Could you check a few things on this model? Use its own coordinates, in mm. A direction names the side the tool comes from. Coordinates: 2 decimals unless noted, no trailing zeros. Loops run counter-clockwise (first coordinate to the right, second up) from the corner with the lowest first, then second, coordinate; pieces in that order, holes last.
from build123d import *

# Parameters (mm, degrees)
F0_R      = 2.0955
F0_R_2    = 4.826
F1_DEPTH  = 12.7
F2_R      = 2.0955
F3_DEPTH  = 15.875
F4_R      = 5.7785
F5_DEPTH  = 1.4478
F6_R      = 2.413
F7_DEPTH  = 31.75
F8_R      = 3.96875
F9_DEPTH  = 4.7498
F10_R     = 1.5875
F10_R_2   = 2.0066
F11_DEPTH = 9.525


with BuildPart() as f1:
    # F0 (on Top) → F1 (new body)
    with BuildSketch(Plane.XY):
        with BuildLine():
            Line((33.3375, -18.796), (33.3375, 18.796))
            Line((33.3375, 18.796), (-33.3375, 18.796))
            Line((-33.3375, 18.796), (-33.3375, 9.9949))
            Line((-33.3375, 9.9949), (-20.271096, 9.9949))
            ThreePointArc((-20.271096, 9.9949), (4.938511, -9.285687), (-21.315194, 8.5471))
            Line((-21.315194, 8.5471), (-33.3375, 8.5471))
            Line((-33.3375, 8.5471), (-33.3375, -18.796))
            Line((-33.3375, -18.796), (33.3375, -18.796))
        make_face()
        with Locations((-21.7805, -13.843)):
            Circle(F0_R, mode=Mode.SUBTRACT)
        with Locations((25.8699, -5.461)):
            Circle(F0_R_2, mode=Mode.SUBTRACT)
        with Locations((6.0325, 13.843)):
            Circle(F0_R, mode=Mode.SUBTRACT)
    extrude(amount=F1_DEPTH)

    # F2 (on face) → F3 (cut)
    with BuildSketch(Plane.YZ.offset(33.3375)):
        with Locations((-13.4874, 6.35)):
            Circle(F2_R)
        with Locations((13.4874, 6.35)):
            Circle(F2_R)
    extrude(amount=-F3_DEPTH, mode=Mode.SUBTRACT)

    # F4 (on face) → F5 (cut)
    with BuildSketch(Plane(origin=(0, 0, 0), x_dir=(1, 0, 0), z_dir=(0, 0, -1))):
        with Locations((25.8699, 5.461)):
            Circle(F4_R)
    extrude(amount=-F5_DEPTH, mode=Mode.SUBTRACT)

    # F6 (on face) → F7 (cut)
    with BuildSketch(Plane(origin=(0, 18.796, 0), x_dir=(-1, 0, 0), z_dir=(0, 1, 0))):
        with Locations((26.9875, 6.35)):
            Circle(F6_R)
    extrude(amount=-F7_DEPTH, mode=Mode.SUBTRACT)

    # F8 (on face) → F9 (cut)
    with BuildSketch(Plane(origin=(0, 18.796, 0), x_dir=(-1, 0, 0), z_dir=(0, 1, 0))):
        with Locations((26.9875, 6.35)):
            Circle(F8_R)
    extrude(amount=-F9_DEPTH, mode=Mode.SUBTRACT)

    # F10 (on face) → F11 (cut)
    with BuildSketch(Plane(origin=(0, 18.796, 0), x_dir=(-1, 0, 0), z_dir=(0, 1, 0))):
        with Locations((19.80565, 6.35)):
            Circle(F10_R)
        with Locations((0.75565, 6.35)):
            Circle(F10_R_2)
    extrude(amount=-F11_DEPTH, mode=Mode.SUBTRACT)


solid = f1.part
(1) Imagine slicing it at B-B, the plane y = 3.5. Write out the boundary of the cut face in (x, z), and give its area (3 significant figures).
Answers:
outline: (-33.34, 0) - (-23.42, 0) - (-23.42, 12.7) - (-33.34, 12.7) - close; (7.55, 0) - (33.34, 0) - (33.34, 12.7) - (7.55, 12.7) - close; hole circle Ø4.83 at (-26.99, 6.35)
area: 435 mm2
(2) Imagine slicing it at A-A, the plane x = 25. Write out the boundary of the cut face in (y, z), and give its area (3 significant figures).
Answers:
outline: (-18.8, 0) - (-11.17, 0) - (-11.17, 1.45) - (-10.21, 1.45) - (-10.21, 12.7) - (-18.8, 12.7) - close; (-0.71, 1.45) - (0.25, 1.45) - (0.25, 0) - (18.8, 0) - (18.8, 12.7) - (-0.71, 12.7) - close; hole circle Ø4.19 at (-13.49, 6.35); hole circle Ø4.19 at (13.49, 6.35)
area: 326 mm2
(3) I need wall thicknesses on probe 1 along X at (y, z) = (2.5, 7); probe 2 along X at (y, z) = (3.5, 8.5); probe 3 along Y at (x, z) = (-8.5, 1.75). Which ranges of each line are inside material? Lowest first, please.
Answers:
probe 1: x = -33.34 to -29.31, -24.66 to -23.61, 7.74 to 33.34
probe 2: x = -33.34 to -28.08, -25.89 to -23.42, 7.55 to 33.34
probe 3: y = -18.8 to -15.87, 15.87 to 18.8
(4) Imagine slicing it at D-D, the plane y = -9.5. Write out the boundary of the cut face in (x, z).
Answers:
outline: (-33.34, 0) - (-20.66, 0) - (-20.66, 12.7) - (-33.34, 12.7) - close; (4.78, 0) - (21.74, 0) - (21.74, 1.45) - (23.23, 1.45) - (23.23, 12.7) - (4.78, 12.7) - close; (28.51, 1.45) - (30, 1.45) - (30, 0) - (33.34, 0) - (33.34, 12.7) - (28.51, 12.7) - close; hole circle Ø4.83 at (-26.99, 6.35)
(5) Which directions (+Z, -Z, +X, -X, +Y, -Y) give clear straight access to the entire face, cutting with the end or side of a thin tool? Please do faces 4 (the face through (31.38, -7.2, 0.71)), 5 (the face through (-30, 14.046, 6)), 6 (the face through (25.5, -15, 7.8)).
Answers:
face 4: -Z
face 5: +Y
face 6: +X
(6) Imagine slicing it at C-C, the plane z = 11. State how many separate pieces and enclosed holes the cut face has, and give its area (3 significant figures).
Answers:
separate pieces: 1
enclosed holes: 3
area: 1,600 mm2
(7) For pin 1 (2.5 mm diameter, centred on x = -28, z = 7, fed in from +Y); pin 2 (6 mm diameter, centred on x = 25.87, y = -5.46, fed in from +Z), each with a flat end and sliding along its axis, tell me the tip position at first contact or that it passes through.
Answers:
pin 1: stops at y = 14.05
pin 2: passes through
(8) We'd pull the mould along Z, two halves only. Please class faces 1 (the face through (7, 9, 0)), 2 (the face through (6.999, 11.984, 6.261)), 3 (the face through (-21.27, 14.46, 5.74)): +Z half, -Z half, draft (parallel to the pull), parting line (faces both ways), or undercut.
Answers:
face 1: -Z half
face 2: draft
face 3: undercut
